```python
from build123d import *

# Parameters (mm, degrees)
F5_R   = 12.5
F5_R_2 = 9.9999973178


with BuildPart() as f8:
    # F8: sweep along a path in F7, F3
    with BuildLine(Plane(origin=(77.5, 0, 0), x_dir=(0, -1, 0), z_dir=(-1, 0, 0))) as f8_path:
        Line((400, 0), (15.7675532053, 0))
        ThreePointArc((15.7675532053, 0), (0.316538288, 1.5558353919), (-14.5141092526, 6.1608738574))
        Line((-14.5141092526, 6.1608738574), (-32.9246175983, 13.9756710038))
    with BuildLine(Plane(origin=(0, 0, 0), x_dir=(1, 0, 0), z_dir=(0, 0.3907311285, -0.9205048535))) as f8_path_2:
        ThreePointArc((77.5, -35.768), (54.800775542, -90.568775542), (0, -113.268))
    # F5 (on plane+point) → F8 (sweep)
    with BuildSketch(Plane.XZ.offset(400)):
        with Locations((77.5, 0)):
            Circle(F5_R)
        with Locations((77.5, 0)):
            Circle(F5_R_2, mode=Mode.SUBTRACT)
    sweep(path=f8_path.line + f8_path_2.line)

    # F9: F8 across plane


with BuildPart() as f8_1:
    add(f8.part)
    add(f8.part.mirror(Plane.YZ))


solid = f8_1.part
```
Check sheet for the modelled part. Datum: model origin and axes. Units: mm. A direction names the side the tool comes from. Round coordinates to 2 decimals unless told otherwise and drop trailing zeros. Order: outer loops, then holes, each group sorted by start corner. A loop starts at its lowest first (then second) coordinate and runs counter-clockwise, first axis right, second up. Notation, with made-up numbers: (-1.5, 78.25) - (44.5, 78.25) arc R14 ccw to (44.5, 85.25) - close; hole circle Ø8 at (-2, -9.5). An arc over 180 degrees is marked (long way). Write item = value, one per line.
Q1. Tool access check on faces 3 (the face through (87.04, -205.19, -3)), 4 (the face through (-65, 24, 10)). Record the directions out of +Z, -Z, +X, -X, +Y, -Y that give a thin tool (end or side, any length) a straight path to the whole face; none if there is none.
Computed:
face_3 = -Y
face_4 = none
Q2. Thickness scan on line 1 along X through (y, z) = (-14.5, 0.5); line 2 along Z through (x, y) = (-77.5, -167); line 3 along X through (y, z) = (-358.5, -4.5). Record the ranges inside material, lowest first.
Computed:
line_1 = -89.99 to -87.49, -67.51 to -65.01, 65.01 to 67.51, 87.49 to 89.99
line_2 = -12.5 to -10, 10 to 12.5
line_3 = -89.16 to -86.43, -68.57 to -65.84, 65.84 to 68.57, 86.43 to 89.16
Q3. Draft check along X on faces 1 (the face through (-65.012, -205.194, -0.55)), 2 (the face through (86, -400, 6)). Enter one of: pulls with the +X half, pulls with the -X half, needs draft (parallel to the pull), parting line crosses it, or undercut.
Computed:
face_1 = undercut
face_2 = needs draft
Q4. Section check A-A (y = -101.5). Record the boundary of the cut face in (x, z), and give its area (3 significant figures).
Computed:
outline = circle Ø25 at (-77.5, 0); circle Ø25 at (77.5, 0); hole circle Ø20 at (-77.5, 0); hole circle Ø20 at (77.5, 0)
area = 353 mm^2
Q5. Go/stop test with flat-tipped pins: pin 1 (10 mm diameter, centred on y = -19, z = 11, fed in from -X); pin 2 (16 mm diameter, centred on x = 77.5, z = 0, fed in from +Y). Record where each tip stops, or that it passes through.
Computed:
pin_1 = -88.47
pin_2 = 50.74
Q6. Section check B-B (y = 64.5). State how many separate pieces and enclosed holes the cut face has, and give its area (3 significant figures).
Computed:
separate_pieces = 2
enclosed_holes = 2
area = 431 mm^2
